```python
from build123d import *

# Parameters (mm, degrees)
BOSS_EXTRUDE1_DEPTH = 4.572
SKETCH3_W           = 115.1315452
SKETCH3_H           = 4.572
BOSS_EXTRUDE2_DEPTH = 17.78
FILLET1_R           = 2.54
SKETCH4_W           = 121.92
SKETCH4_H           = 19.304
BOSS_EXTRUDE4_DEPTH = 5.08
SKETCH5_W           = 12.7
SKETCH5_H           = 6.35
CUT_EXTRUDE1_DEPTH  = 5.08
SKETCH6_R           = 1.27
CUT_EXTRUDE2_DEPTH  = 6.35


with BuildPart() as part:
    # Sketch2 → Boss-Extrude1 (new body)
    with BuildSketch(Plane(origin=(0, 0, 0), x_dir=(-1, 0, 0), z_dir=(0, 0, -1))):
        with BuildLine():
            Line((-62.487415839, 48.848476089), (52.644129361, 48.848476089))
            Line((52.644129361, 48.848476089), (41.713156468, -49.932022311))
            ThreePointArc((41.713156468, -49.932022311), (40.052782988, -53.157778108), (36.663977171, -54.453284069))
            Line((36.663977171, -54.453284069), (-46.507263649, -54.453284069))
            ThreePointArc((-46.507263649, -54.453284069), (-49.896069466, -53.157778108), (-51.556442946, -49.932022311))
            Line((-51.556442946, -49.932022311), (-62.487415839, 48.848476089))
        make_face()
    extrude(amount=BOSS_EXTRUDE1_DEPTH)

    # Sketch3 → Boss-Extrude2 (add)
    with BuildSketch(Plane(origin=(0, 48.848476089, 0), x_dir=(1, 0, 0), z_dir=(0, 1, 0))):
        with Locations((4.921643239, 2.286)):
            Rectangle(SKETCH3_W, SKETCH3_H)
    extrude(amount=BOSS_EXTRUDE2_DEPTH)

    # Fillet1
    fillet1_edges = [part.edges().sort_by_distance(p)[0] for p in [
        (62.487415839, 48.848476089, -2.286),
        (-52.644129361, 48.848476089, -2.286),
    ]]
    fillet(fillet1_edges, radius=FILLET1_R)

    # Sketch4 → Boss-Extrude4 (add)
    with BuildSketch(Plane(origin=(0, 66.628476089, 0), x_dir=(1, 0, 0), z_dir=(0, 1, 0))):
        with Locations((4.921643239, 2.286)):
            Rectangle(SKETCH4_W, SKETCH4_H)
    extrude(amount=BOSS_EXTRUDE4_DEPTH)

    # Sketch5 → Cut-Extrude1 (cut)
    with BuildSketch(Plane(origin=(0, 0, -4.572), x_dir=(-1, 0, 0), z_dir=(0, 0, -1))):
        with Locations((-4.921643239, -38.578284069)):
            Rectangle(SKETCH5_W, SKETCH5_H)
    extrude(amount=-CUT_EXTRUDE1_DEPTH, mode=Mode.SUBTRACT)

    # Sketch6 → Cut-Extrude2 (cut)
    with BuildSketch(Plane(origin=(0, 0, -4.572), x_dir=(-1, 0, 0), z_dir=(0, 0, -1))):
        Polygon((10.078356761, -23.771523911), (10.078356761, 36.228476089), (5.078356761, 36.228476089), (5.078356761, 41.228476089), (-14.921643239, 41.228476089), (-14.921643239, 36.228476089), (-19.921643239, 36.228476089), (-19.921643239, -23.771523911), (-14.921643239, -23.771523911), (-14.921643239, -28.771523911), (5.078356761, -28.771523911), (5.078356761, -23.771523911), align=None)
        with Locations((-17.421643239, 38.728476089)):
            Circle(SKETCH6_R)
        with Locations((7.578356761, -26.271523911)):
            Circle(SKETCH6_R)
        with Locations((-17.421643239, -26.271523911)):
            Circle(SKETCH6_R)
        with Locations((-22.421643239, -31.311523911)):
            Circle(SKETCH6_R)
        with Locations((12.578356761, -31.311523911)):
            Circle(SKETCH6_R)
        with Locations((12.578356761, 43.768476089)):
            Circle(SKETCH6_R)
        with Locations((-22.421643239, 43.768476089)):
            Circle(SKETCH6_R)
        with Locations((7.578356761, 38.728476089)):
            Circle(SKETCH6_R)
    extrude(amount=-CUT_EXTRUDE2_DEPTH, mode=Mode.SUBTRACT)


solid = part.part
```
CAD build for the part. Positions are in the model's coordinates, mm. A direction names the side the tool comes from. Round coordinates to 2 decimals unless told otherwise and drop trailing zeros. Order: outer loops, then holes, each group sorted by start corner. A loop starts at its lowest first (then second) coordinate and runs counter-clockwise, first axis right, second up.
Q1. Slice it at D-D (y = 6.5). Write the cut outline in (x, z), and give its area (3 significant figures).
Q2. Slice it at B-B (y = -11). Write the cut outline in (x, z), and give its area (3 significant figures).
Q3. Two-plate mould, pull along Y, no slides. Class faces 5 (the flat face through (4, 71.708, -2)), 6 (the flat face through (4, 69, -11.938)), 7 (the flat face through (-8, 36.228, -2)): pulls with the +Y half, pulls with the -Y half, needs draft (parallel to the pull), parting line crosses it, or undercut.
Q4. Slice it at C-C (x = -26.5). Write the cut outline in (y, z), and give its area (3 significant figures).
Q5. Wall check: L1, parallel to Y at x = 49, z = -9.25; L2, parallel to Z at x = -20, y = 60; L3, parallel to X at y = 54.5, z = -2.5. Give the ranges that are in metal, low to high.
Q6. Slice it at A-A (x = 3). Write the cut outline in (y, z), and give its area (3 significant figures).
Q7. Drop flat-ended pins along their axis: pin 1 (3 mm diameter, centred on y = 4.5, z = -5.5, fed in from -X); pin 2 (1.5 mm diameter, centred on x = -7.58, y = 38.73, fed in from +Z); pin 3 (2.5 mm diameter, centred on y = 59.5, z = -1, fed in from -X); pin 4 (10 mm diameter, centred on y = 48.5, z = -6, fed in from +X). Give the stop position or say it passes through.
Q8. Which spindle directions (+Z, -Z, +X, -X, +Y, -Y) get a long thin tool onto all of the face, cutting with end or side? Do faces 1 (the flat face through (4, 69, 7.366)), 2 (the flat face through (62.487, 58, -2)), 3 (the flat face through (30, 5, -4.572)), 4 (the flat face through (14.922, -26, -2)). Say none if no direction does.
Results below:
1. outline: (-47.96, -4.57) - (-10.08, -4.57) - (-10.08, 0) - (-47.96, 0) - close; (19.92, -4.57) - (57.8, -4.57) - (57.8, 0) - (19.92, 0) - close
1. area: 346 mm2
2. outline: (-46.02, -4.57) - (-10.08, -4.57) - (-10.08, 0) - (-46.02, 0) - close; (19.92, -4.57) - (55.86, -4.57) - (55.86, 0) - (19.92, 0) - close
2. area: 329 mm2
3. face 5: pulls with the +Y half
3. face 6: needs draft
3. face 7: undercut
4. outline: (-54.45, -4.57) - (66.63, -4.57) - (66.63, -11.94) - (71.71, -11.94) - (71.71, 7.37) - (66.63, 7.37) - (66.63, 0) - (-54.45, 0) - close
4. area: 652 mm2
5. L1: y = 66.63 to 71.71
5. L2: z = -4.57 to 0
5. L3: x = -52.64 to 62.49
6. outline: (-54.45, -4.57) - (-41.75, -4.57) - (-41.75, 0) - (-54.45, 0) - close; (-35.4, -4.57) - (-28.77, -4.57) - (-28.77, 0) - (-35.4, 0) - close; (41.23, -4.57) - (66.63, -4.57) - (66.63, -11.94) - (71.71, -11.94) - (71.71, 7.37) - (66.63, 7.37) - (66.63, 0) - (41.23, 0) - close
6. area: 303 mm2
7. pin 1: stops at x = -47.87
7. pin 2: passes through
7. pin 3: stops at x = -52.64
7. pin 4: stops at x = 62.49
8. face 1: +Z, +X, -X, +Y, -Y
8. face 2: +Z, -Z, +X, -Y
8. face 3: -Z, +X, -X, -Y
8. face 4: +Z, -Z
